```python
from build123d import *

# Parameters (mm, degrees)
ESQUISSE2_W                                    = 72
ESQUISSE2_H                                    = 14
BOSS_EXTRU_1_DEPTH                             = 41
ESQUISSE12_W                                   = 9
ESQUISSE12_H                                   = 20
BOSS_EXTRU_6_DEPTH                             = 14
FRAISAGE_POUR_VIS_T_TE_FRAIS_E_M41_D           = 4.3
FRAISAGE_POUR_VIS_T_TE_FRAIS_E_M41_CSINK_D     = 9.4
FRAISAGE_POUR_VIS_T_TE_FRAIS_E_M41_CSINK_ANGLE = 90
ENL_V_MAT_EXTRU_3_REACH                        = 95.798
ESQUISSE6_W                                    = 20
ESQUISSE6_H                                    = 10
ESQUISSE5_W                                    = 5.5
ESQUISSE5_H                                    = 50
ENL_V_MAT_EXTRU_2_DEPTH                        = 7
CHANFREIN1_SIZE                                = 2
ESQUISSE16_W                                   = 20
ESQUISSE16_H                                   = 7
BOSS_EXTRU_7_DEPTH                             = 10
CONG_1_R                                       = 3


with BuildPart() as part:
    # Esquisse2 → Boss.-Extru.1 (new, symmetric)
    with BuildSketch(Plane.XY):
        Rectangle(ESQUISSE2_W, ESQUISSE2_H)
    extrude(amount=BOSS_EXTRU_1_DEPTH, both=True)

    # Esquisse12 → Boss.-Extru.6 (add)
    with BuildSketch(Plane(origin=(0, 7, 0), x_dir=(1, 0, 0), z_dir=(0, 1, 0))):
        with Locations((40.5, 0)):
            Rectangle(ESQUISSE12_W, ESQUISSE12_H)
    extrude(amount=-BOSS_EXTRU_6_DEPTH)

    # Fraisage pour vis à tête fraisée M41 (through all)
    with Locations(Plane(origin=(0, 7, 0), x_dir=(1, 0, 0), z_dir=(0, 1, 0))):
        with Locations((32.5, 0), (7.5, 0)):
            CounterSinkHole(FRAISAGE_POUR_VIS_T_TE_FRAIS_E_M41_D / 2, FRAISAGE_POUR_VIS_T_TE_FRAIS_E_M41_CSINK_D / 2, counter_sink_angle=FRAISAGE_POUR_VIS_T_TE_FRAIS_E_M41_CSINK_ANGLE)

    # Esquisse6 → Enlèv. mat.-Extru.3 (cut, up to next)
    with BuildSketch(Plane.XY.offset(-41), mode=Mode.PRIVATE) as enl_v_mat_extru_3_sk1:
        with Locations((-18, -2)):
            Rectangle(ESQUISSE6_W, ESQUISSE6_H)
    enl_v_mat_extru_3_tool1 = extrude(enl_v_mat_extru_3_sk1.sketch, amount=ENL_V_MAT_EXTRU_3_REACH, mode=Mode.PRIVATE) & part.part
    add(enl_v_mat_extru_3_tool1.solids().sort_by_distance((-18, -2, -41))[0], mode=Mode.SUBTRACT)

    # Esquisse5 → Enlèv. mat.-Extru.2 (cut)
    with BuildSketch(Plane(origin=(0, -7, 0), x_dir=(1, 0, 0), z_dir=(0, 1, 0))):
        with Locations((-33.25, 0)):
            Rectangle(ESQUISSE5_W, ESQUISSE5_H)
    extrude(amount=ENL_V_MAT_EXTRU_2_DEPTH, mode=Mode.SUBTRACT)

    # Chanfrein1
    chanfrein1_edges = [part.edges().sort_by_distance(p)[0] for p in [
        (0, 7, -41),
        (0, 7, 41),
    ]]
    chamfer(chanfrein1_edges, length=CHANFREIN1_SIZE)

    # Esquisse16 → Boss.-Extru.7 (add)
    with BuildSketch(Plane.XZ.offset(-3)):
        with Locations((-18, -37.5)):
            Rectangle(ESQUISSE16_W, ESQUISSE16_H)
    boss_extru_7 = extrude(amount=BOSS_EXTRU_7_DEPTH)

    # Symétrie1: Boss.-Extru.7 across plane
    add(boss_extru_7.mirror(Plane.XY))

    # Congé1
    cong_1_edges = [part.edges().sort_by_distance(p)[0] for p in [
        (45, 0, 10),
        (45, 0, -10),
    ]]
    fillet(cong_1_edges, radius=CONG_1_R)


solid = part.part
```
The model under review builds one solid part; all positions refer to its coordinate system, in mm. A direction names the side the tool comes from. Round coordinates to 2 decimals unless told otherwise and drop trailing zeros. Loops run counter-clockwise (first coordinate to the right, second up) from the corner with the lowest first, then second, coordinate; pieces in that order, holes last.
1) The part is to be moulded in two halves that separate along Z. For faces 5 (the face through (39, 0, -10)), 6 (the face through (-18, -2, -34)), 7 (the face through (44.14, -0.1, 9.1)), 8 (the face through (13, -7, -1)), say which applies: pulls with the +Z half, pulls with the -Z half, needs draft (parallel to the pull), parting line crosses it, or undercut.
Values follow:
face 5: pulls with the -Z half
face 6: undercut
face 7: pulls with the +Z half
face 8: needs draft
2) Clearance check with flat-ended pins moving along their axes: P1, Ø3, axis at x = 40.5, y = 1.5, coming from the +Z side; P2, Ø5, axis at y = -3, z = 14, coming from the +X side; P3, Ø1.6, axis at x = -34.5, z = 5.5, coming from the -Y side. State where each tip first meets the part, or that it passes through.
Values follow:
P1: stops at z = 10
P2: stops at x = 36
P3: stops at y = 0
3) Consider section B-B on y = -4. State the section outline as (x, z) points.
Values follow:
outline: (-36, -41) - (36, -41) - (36, -10) - (42, -10) arc R3 ccw to (45, -7) - (45, 7) arc R3 ccw to (42, 10) - (36, 10) - (36, 41) - (-36, 41) - (-36, 25) - (-30.5, 25) - (-30.5, -25) - (-36, -25) - close; hole (-28, -34) - (-8, -34) - (-8, 34) - (-28, 34) - close; hole circle Ø4.3 at (7.5, 0); hole circle Ø4.3 at (32.5, 0)
4) Consider section D-D on x = -12. State the section outline as (y, z) points, then the cut area to 3 significant figures.
Values follow:
outline: (-7, -41) - (5, -41) - (7, -39) - (7, 39) - (5, 41) - (-7, 41) - (-7, 34) - (3, 34) - (3, -34) - (-7, -34) - close
area: 464 mm2
5) Consider section A-A on x = 32.5. State the section outline as (y, z) points.
Values follow:
outline: (-7, -41) - (5, -41) - (7, -39) - (7, -4.7) - (4.45, -2.15) - (-7, -2.15) - close; (-7, 2.15) - (4.45, 2.15) - (7, 4.7) - (7, 39) - (5, 41) - (-7, 41) - close
6) Wall thickness on line 1 along Z through (x, y) = (7.5, 0.75); line 2 along X through (y, z) = (-5, -23); line 3 along Z through (x, y) = (-22.5, -0.25): over which ranges is each line inside the solid? List them lowest first.
Values follow:
line 1: z = -41 to -2.15, 2.15 to 41
line 2: x = -30.5 to -28, -8 to 36
line 3: z = -41 to -34, 34 to 41
7) Consider section C-C on z = 0. State the section outline as (x, y) points.
Values follow:
outline: (-36, 0) - (-30.5, 0) - (-30.5, -7) - (-28, -7) - (-28, 3) - (-8, 3) - (-8, -7) - (5.35, -7) - (5.35, 4.45) - (2.8, 7) - (-36, 7) - close; (9.65, -7) - (30.35, -7) - (30.35, 4.45) - (27.8, 7) - (12.2, 7) - (9.65, 4.45) - close; (34.65, -7) - (45, -7) - (45, 7) - (37.2, 7) - (34.65, 4.45) - close
8) Tool access review of faces 1 (the face through (36, 0, -25)), 2 (the face through (-33, 0, 0)), 3 (the face through (-28, -2, 0)), 4 (the face through (39, 0, 10)): name each direction out of +Z, -Z, +X, -X, +Y, -Y from which nothing blocks a thin tool from reaching the whole face with its end or side.
Values follow:
face 1: -Z, +X, +Y, -Y
face 2: -X, -Y
face 3: -Y
face 4: +Z, +X, +Y, -Y
